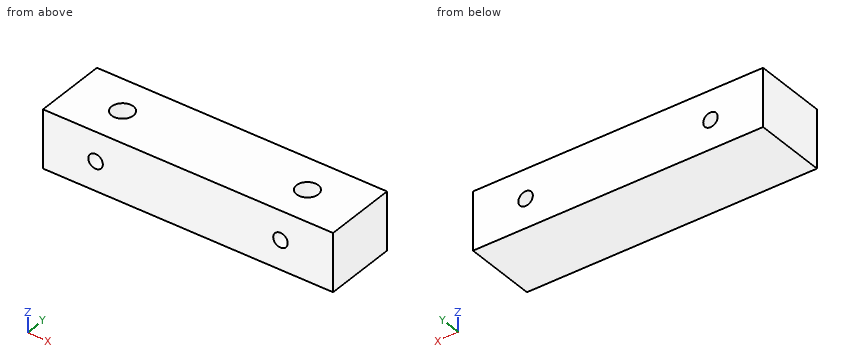
from build123d import *

# Parameters (mm, degrees)
F0_W     = 254
F0_H     = 50.8
F1_DEPTH = 31.75
F2_R     = 9.525
F3_DEPTH = 44.45
F4_R     = 6.35
F5_DEPTH = 63.501


with BuildPart() as f1:
    # F0 (on Front) → F1 (new body, symmetric)
    with BuildSketch(Plane.XZ):
        Rectangle(F0_W, F0_H)
    extrude(amount=F1_DEPTH, both=True)

    # F2 (on face) → F3 (cut)
    with BuildSketch(Plane.XY.offset(25.4)):
        with Locations((-80.9498, 0)):
            Circle(F2_R)
        with Locations((80.9498, 0)):
            Circle(F2_R)
    extrude(amount=-F3_DEPTH, mode=Mode.SUBTRACT)

    # F4 (on face) → F5 (cut, through all)
    with BuildSketch(Plane.XZ.offset(31.75)):
        with Locations((-80.9498, 0)):
            Circle(F4_R)
        with Locations((80.9498, 0)):
            Circle(F4_R)
    extrude(amount=-F5_DEPTH, mode=Mode.SUBTRACT)


solid = f1.part
Check sheet for the modelled part. Datum: model origin and axes. Units: mm. Round coordinates to 2 decimals unless told otherwise and drop trailing zeros. Loops run counter-clockwise (first coordinate to the right, second up) from the corner with the lowest first, then second, coordinate; pieces in that order, holes last.
1. Scan lines: probe 1 along X at (y, z) = (-21, 0); probe 2 along X at (y, z) = (-15, -4.5); probe 3 along Z at (x, y) = (73, -2). Record each from-to range of solid material in increasing order.
2. Sectioned sample at D-D on y = 14. Record the boundary of the cut face in (x, z), and give its area (3 significant figures).
3. Sectioned sample at B-B on z = 12.5. Record the boundary of the cut face in (x, y) (3 decimals), and give its area (3 significant figures).
4. Gauge pin test, flat end, axial feed: pin 1 Ø5.5 at (x, y) = (76.5, -4.5) entering from +Z. Record the tip position at first contact, or that the pin passes through.
5. Sectioned sample at C-C on y = 0. Record the boundary of the cut face in (x, z).
6. Sectioned sample at A-A on z = 0. Record the boundary of the cut face in (x, y) (3 decimals), and give its area (3 significant figures).
Recorded:
1. probe 1: x = -127 to -87.3, -74.6 to 74.6, 87.3 to 127
1. probe 2: x = -127 to -85.43, -76.47 to 76.47, 85.43 to 127
1. probe 3: z = -25.4 to -19.05
2. outline: (-127, -25.4) - (127, -25.4) - (127, 25.4) - (-127, 25.4) - close; hole circle Ø12.7 at (-80.95, 0); hole circle Ø12.7 at (80.95, 0)
2. area: 12,600 mm2
3. outline: (-127, -31.75) - (127, -31.75) - (127, 31.75) - (-127, 31.75) - close; hole circle Ø19.05 at (-80.95, 0); hole circle Ø19.05 at (80.95, 0)
3. area: 15,600 mm2
4. pin 1: stops at z = -19.05
5. outline: (-127, -25.4) - (127, -25.4) - (127, 25.4) - (90.47, 25.4) - (90.47, -19.05) - (71.42, -19.05) - (71.42, 25.4) - (-71.42, 25.4) - (-71.42, -19.05) - (-90.47, -19.05) - (-90.47, 25.4) - (-127, 25.4) - close
6. outline: (-127, -31.75) - (-87.3, -31.75) - (-87.3, -7.1) arc R9.525 cw to (-87.3, 7.1) - (-87.3, 31.75) - (-127, 31.75) - close; (-74.6, -31.75) - (74.6, -31.75) - (74.6, -7.1) arc R9.525 cw to (74.6, 7.1) - (74.6, 31.75) - (-74.6, 31.75) - (-74.6, 7.1) arc R9.525 cw to (-74.6, -7.1) - close; (87.3, -31.75) - (127, -31.75) - (127, 31.75) - (87.3, 31.75) - (87.3, 7.1) arc R9.525 cw to (87.3, -7.1) - close
6. area: 14,400 mm2
